The listing builds one solid part. Answer for the finished solid, in the listing's coordinates (mm). A direction names the side the tool comes from. Give positions to 0.01 mm unless a question says otherwise; leave off trailing zeros. Order: outer loops, then holes, each group sorted by start corner. A loop starts at its lowest first (then second) coordinate and runs counter-clockwise, first axis right, second up. Notation, with made-up numbers: (26, -31.5) - (40, -31.5) arc R20 ccw to (40, 5.5) - close; hole circle Ø8 at (-35, 36.5). An arc over 180 degrees is marked (long way). Use a Markdown table: item, result. Add a question column.
1) Straight lines are drawn through the part: line 1 (Y direction, x = 0, z = 52); line 2 (Y direction, x = 0, z = 8); line 3 (Z direction, x = 23, y = 9.5). For each, find the intervals that lie inside material, in ascending order.
2) Flat-ended cylindrical pins translate along their axes: pin 1 (4.5 mm diameter, centred on x = 24, y = 0, fed in from -Z); pin 2 (5.5 mm diameter, centred on x = -0.5, z = 14.5, fed in from +Y); pin 3 (3 mm diameter, centred on x = 11, y = -6, fed in from -Z); pin 4 (5 mm diameter, centred on x = -0.5, y = 2, fed in from -Z). Find the tip coordinate at first contact, or state that the pin passes through.
3) Find section C-C, the plane z = 17. Determine the outline of the cut face in (x, y), plus the area to 3 significant figures.
4) For faces 1 (the face through (-2.5, 6, 11)), 2 (the face through (-22.35, 0.07, 51.52)), 3 (the face through (4.1, -8.3, 44.05)), determine the directions among +Z, -Z, +X, -X, +Y, -Y from which every point of the face is accessible in a straight line to the end or side of a thin tool.
5) The mould has two halves that part along Y. Classify faces 4 (the face through (0.215, -22.364, 51.515)), 5 (the face through (0, 5, 11)), 6 (the face through (0, -3, 2)): released by +Y, released by -Y, zero draft, split by the parting line, or undercut.
6) Find section A-A, the plane x = 24. Determine the outline of the cut face in (y, z).
7) Find section D-D, the plane y = 18. Determine the outline of the cut face in (x, z), plus the area to 3 significant figures.
from build123d import *

# Parameters (mm, degrees)
SKETCH1_R                 = 7.5
BOSS_EXTRUDE1_DEPTH       = 20.05
SKETCH3_W                 = 5
SKETCH3_H                 = 5
CUT_EXTRUDE1_DEPTH        = 21
SKETCH6_R                 = 8.5
BOSS_EXTRUDE2_DEPTH       = 24
SKETCH7_R                 = 11.25
BOSS_EXTRUDE3_DEPTH       = 5
SKETCH8_R                 = 30
BOSS_EXTRUDE4_DEPTH       = 5
FILLET1_R                 = 0.6
FILLET2_R                 = 5
M4X0_7_TAPPED_HOLE1_D     = 3.3
M6X1_0_TAPPED_HOLE2_D     = 5
M6X1_0_TAPPED_HOLE2_DEPTH = 23.497848452
M6X1_0_TAPPED_HOLE2_TIP   = 1.502151548
SKETCH13_R                = 7.5
CUT_EXTRUDE2_DEPTH        = 2


with BuildPart() as part:
    # Sketch1 → Boss-Extrude1 (new body)
    with BuildSketch(Plane.XY):
        Circle(SKETCH1_R)
    extrude(amount=BOSS_EXTRUDE1_DEPTH)

    # Sketch3 → Cut-Extrude1 (cut)
    with BuildSketch(Plane(origin=(0, 0, 0), x_dir=(-1, 0, 0), z_dir=(0, 0, -1))):
        with Locations((0, 7.5)):
            Rectangle(SKETCH3_W, SKETCH3_H)
    extrude(amount=-CUT_EXTRUDE1_DEPTH, mode=Mode.SUBTRACT)

    # Sketch6 → Boss-Extrude2 (add)
    with BuildSketch(Plane.XY.offset(20.05)):
        Circle(SKETCH6_R)
    extrude(amount=BOSS_EXTRUDE2_DEPTH)

    # Sketch7 → Boss-Extrude3 (add)
    with BuildSketch(Plane.XY.offset(44.05)):
        Circle(SKETCH7_R)
    extrude(amount=BOSS_EXTRUDE3_DEPTH)

    # Sketch8 → Boss-Extrude4 (add)
    with BuildSketch(Plane.XY.offset(49.05)):
        Circle(SKETCH8_R)
    extrude(amount=BOSS_EXTRUDE4_DEPTH)

    # Fillet1
    fillet1_edges = [part.edges().sort_by_distance(p)[0] for p in [
        (-8.5, 0, 44.05),
    ]]
    fillet(fillet1_edges, radius=FILLET1_R)

    # Fillet2
    fillet2_edges = [part.edges().sort_by_distance(p)[0] for p in [
        (-11.25, 0, 49.05),
    ]]
    fillet(fillet2_edges, radius=FILLET2_R - 0.0001)  # a hair under: the kernel refuses the full size

    # M4x0.7 Tapped Hole1 (through all)
    with Locations(Plane.XY.offset(54.05)):
        with Locations((0, 24), (0, -24), (24, 0), (-24, 0)):
            Hole(M4X0_7_TAPPED_HOLE1_D / 2)

    # M6x1.0 Tapped Hole2
    with Locations(Plane(origin=(0, 0, 0), x_dir=(-1, 0, 0), z_dir=(0, 0, -1))):
        with Locations((0, 0)):
            Hole(M6X1_0_TAPPED_HOLE2_D / 2, depth=M6X1_0_TAPPED_HOLE2_DEPTH)
            with Locations((0, 0, -(M6X1_0_TAPPED_HOLE2_DEPTH + M6X1_0_TAPPED_HOLE2_TIP / 2))):  # 118° drill point
                Cone(0, M6X1_0_TAPPED_HOLE2_D / 2, M6X1_0_TAPPED_HOLE2_TIP, mode=Mode.SUBTRACT)

    # Sketch13 → Cut-Extrude2 (cut)
    with BuildSketch(Plane(origin=(0, 0, 0), x_dir=(-1, 0, 0), z_dir=(0, 0, -1))):
        Circle(SKETCH13_R)
    extrude(amount=-CUT_EXTRUDE2_DEPTH, mode=Mode.SUBTRACT)


solid = part.part
The answers:
| question | item | result |
|---|---|---|
| 1 | line 1 | -30 to -25.65, -22.35 to 22.35, 25.65 to 30 |
| 1 | line 2 | -7.5 to -2.5, 2.5 to 5 |
| 1 | line 3 | 49.05 to 54.05 |
| 2 | pin 1 | z = 49.05 |
| 2 | pin 2 | y = 7.07 |
| 2 | pin 3 | z = 44.05 |
| 2 | pin 4 | z = 2 |
| 3 | outline | (-2.5, 5) - (-2.5, 7.07) arc R7.5 ccw (long way) to (2.5, 7.07) - (2.5, 5) - close; hole circle Ø5 at (0, 0) |
| 3 | area | 145 mm2 |
| 4 | face 1 | -Z, +Y |
| 4 | face 2 | +Z, -Z |
| 4 | face 3 | -Z |
| 5 | face 4 | undercut |
| 5 | face 5 | released by +Y |
| 5 | face 6 | zero draft |
| 6 | outline | (-18, 49.05) - (-1.65, 49.05) - (-1.65, 54.05) - (-18, 54.05) - close; (1.65, 49.05) - (18, 49.05) - (18, 54.05) - (1.65, 54.05) - close |
| 7 | outline | (-24, 49.05) - (24, 49.05) - (24, 54.05) - (-24, 54.05) - close |
| 7 | area | 240 mm2 |
